Study the drawing (mm; zero at the part's minimum x, y, z) and answer. A direction names the side the tool comes from. Coordinates: 2 decimals unless noted, no trailing zeros. Write each loop counter-clockwise with the first axis right and the second up, starting at its lowest first coordinate (ties: lowest second). Pieces come first, ordered by that corner, then holes. Notation, with made-up numbers: (-20, 5) -> (0, 5) arc R22 cw to (0, 26) -> close; hole circle Ø4 at (34.5, 22). An arc over 180 degrees is marked (long way). Write item = value, one per line. Start each with the question number.
1) Section D-D (x = 2) is taken. Determine the outline of the cut face in (y, z), plus the area to 3 significant figures.
2) Section C-C (y = 11.5) is taken. Determine the outline of the cut face in (x, z), plus the area to 3 significant figures.
3) A tool of negligible diameter and unlimited length cuts with its end or side. For the marked faces 4, 5, 6, 7 and 8, from which of +Z, -Z, +X, -X, +Y, -Y can it reach the whole face along a straight path? Write none if from no direction.
4) Find the intervals of material crossed by line 1 along X through (y, z) = (9.25, 11); line 2 along X through (y, z) = (6.5, 5.5); line 3 along Z through (x, y) = (9.5, 11), in increasing order. Write a range as from..to.
5) Flat-ended cylindrical pins translate along their axes: pin 1 Ø2 at (x, y) = (8, 8) entering from +Z; pin 2 Ø3 at (x, y) = (5, 2) entering from +Z; pin 3 Ø1 at (x, z) = (4.5, 6.5) entering from -Y. Find the tip coordinate at first contact, or state that the pin passes through.
6) Section B-B (x = 4.25) is taken. Determine the outline of the cut face in (y, z), plus the area to 3 significant figures.
7) Section A-A (z = 11.5) is taken. Determine the outline of the cut face in (x, y), plus the area to 3 significant figures.
8) For a pull along X with two mould halves and no side action, classify the marked faces 1, 2 and 3 as released by +X, released by -X, zero draft, split by the parting line, or undercut.
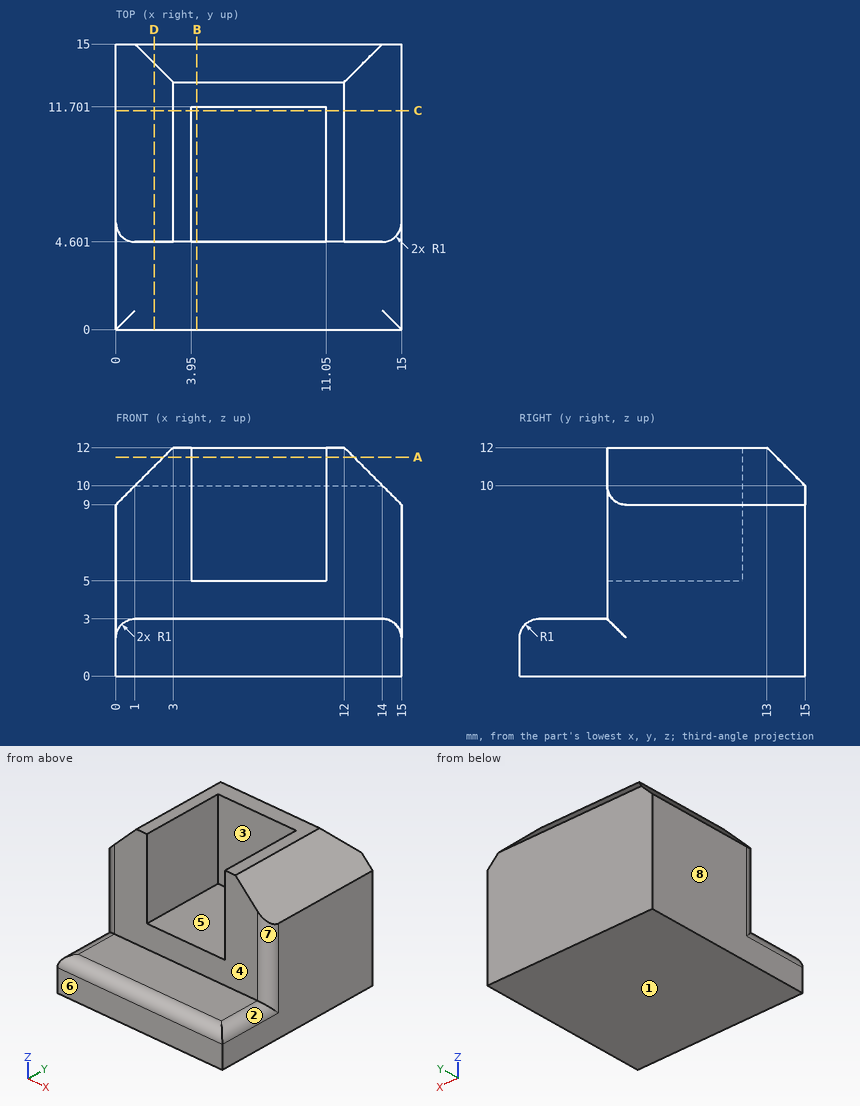
Answer key:
q1.outline = (0, 0) -> (15, 0) -> (15, 10) -> (14, 11) -> (4.6, 11) -> (4.6, 3) -> (1, 3) arc R1 ccw to (0, 2) -> close
q1.area = 127 mm^2
q2.outline = (0, 0) -> (15, 0) -> (15, 9) -> (12, 12) -> (11.05, 12) -> (11.05, 5) -> (3.95, 5) -> (3.95, 12) -> (3, 12) -> (0, 9) -> close
q2.area = 121 mm^2
q3.face_4 = +Z, +X, -X, -Y
q3.face_5 = +Z, -Y
q3.face_6 = +Z, -Z, +X, -X, -Y
q3.face_7 = +Z, +X, -Y
q3.face_8 = +Z, -Z, -X, +Y, -Y
q4.line_1 = 2..3.95, 11.05..13
q4.line_2 = 0..3.95, 11.05..15
q4.line_3 = 0..5
q5.pin_1 = 5
q5.pin_2 = 3
q5.pin_3 = 11.7
q6.outline = (0, 0) -> (15, 0) -> (15, 10) -> (13, 12) -> (11.7, 12) -> (11.7, 5) -> (4.6, 5) -> (4.6, 3) -> (1, 3) arc R1 ccw to (0, 2) -> close
q6.area = 86.7 mm^2
q7.outline = (2.5, 4.6) -> (3.95, 4.6) -> (3.95, 11.7) -> (11.05, 11.7) -> (11.05, 4.6) -> (12.5, 4.6) -> (12.5, 13.5) -> (2.5, 13.5) -> close
q7.area = 38.6 mm^2
q8.face_1 = zero draft
q8.face_2 = released by +X
q8.face_3 = undercut
